Build history of the part. All positions in model axes, mm. A direction names the side the tool comes from. Give positions to 0.01 mm unless a question says otherwise; leave off trailing zeros. Write each loop counter-clockwise with the first axis right and the second up, starting at its lowest first coordinate (ties: lowest second). Pieces come first, ordered by that corner, then holes. Notation, with made-up numbers: M -29,0.5 L -16,0.5 A19 ccw -16,4.5 Z; hole C 84.5,-34 d11. An arc over 180 degrees is marked long. Return JSON: item names as keys, results as strings. Group by question number.
Q1. Band-saw the part on C-C, the plane y = 290. Give the cut face in (x, z) (3 decimals).
Q2. Band-saw the part on A-A, the plane x = -56.5. Give the cut face in (y, z) (3 decimals).
Q3. Pull direction Z, two halves, no side cores. Call faces 1 (the flat face through (-184.15, 279, 100)), 2 (the flat face through (-3, 279, -22.225)), 3 (the flat face through (-190.5, 280, 100)), 4 (the flat face through (-3, 280, 228.6)): +Z half, -Z half, draft (parallel to the pull), parting line (faces both ways), or undercut.
Q4. Tool access for faces 5 (the flat face through (-184.3, 254, 102.2)), 6 (the flat face through (-3, 279, 225.425)): list every direction of +Z, -Z, +X, -X, +Y, -Y with a clear straight run to the whole face (end or side of a thin tool).
Q5. Wall check: probe 1 along Z at (x, y) = (-156, 275) (3 decimals); probe 2 along X at (y, z) = (294, 73.5). Give the ranges that are in metal, low to high.
Q6. Band-saw the part on B-B, the plane z = 58.5. Give the cut face in (x, y).
from build123d import *

# Parameters (mm, degrees)
F0_W     = 381
F0_H     = 254
F1_DEPTH = 50.8
F2_R     = 6.35
F3_R     = 6.35
F5_W     = 368.3
F5_H     = 247.65
F6_DEPTH = 50.8
F7_R     = 3.175


with BuildPart() as f1:
    # F0 (on Front) → F1 (new body)
    with BuildSketch(Plane.XZ):
        Rectangle(F0_W, F0_H)
    extrude(amount=F1_DEPTH)

    # F2
    f2_edges = [f1.edges().sort_by_distance(p)[0] for p in [
        (190.5, -25.4, 127),
    ]]
    fillet(f2_edges, radius=F2_R)

    # F3
    f3_edges = [f1.edges().sort_by_distance(p)[0] for p in [
        (190.5, -25.4, -127),
        (-190.5, -25.4, 127),
        (-190.5, -25.4, -127),
    ]]
    fillet(f3_edges, radius=F3_R)


with BuildPart() as f1_1:
    # F4: moved
    add(f1.part.moved(Location((0, 50.8, 0))))

    # F5 (on Front) → F6 (cut)
    with BuildSketch(Plane.XZ):
        Rectangle(F5_W, F5_H)
    extrude(amount=-F6_DEPTH, mode=Mode.SUBTRACT)

    # F7
    f7_edges = [f1_1.edges().sort_by_distance(p)[0] for p in [
        (184.15, 25.4, -123.825),
        (184.15, 25.4, 123.825),
        (-184.15, 25.4, 123.825),
        (-184.15, 25.4, -123.825),
    ]]
    fillet(f7_edges, radius=F7_R)


with BuildPart() as f1_2:
    # F8: moved
    add(f1_1.part.moved(Location((0, 50.8, 0))))


with BuildPart() as f1_3:
    # F9: moved
    add(f1_2.part.moved(Location((0, 0, -101.6))))


with BuildPart() as f1_4:
    # F10: moved
    add(f1_3.part.moved(Location((0, 203.2, 0))))


with BuildPart() as f1_5:
    # F11: moved
    add(f1_4.part.moved(Location((0, 0, 203.2))))


solid = f1_5.part
From the geometry:
{
 "1": {"outline": "M -190.5,-19.05 A6.35 ccw -184.15,-25.4 L 184.15,-25.4 A6.35 ccw 190.5,-19.05 L 190.5,222.25 A6.35 ccw 184.15,228.6 L -184.15,228.6 A6.35 ccw -190.5,222.25 Z; hole M -184.15,-19.05 A3.175 ccw -180.975,-22.225 L 180.975,-22.225 A3.175 ccw 184.15,-19.05 L 184.15,222.25 A3.175 ccw 180.975,225.425 L -180.975,225.425 A3.175 ccw -184.15,222.25 Z"},
 "2": {"outline": "M 254,-25.4 L 304.8,-25.4 L 304.8,-22.225 L 254,-22.225 Z; M 254,225.425 L 304.8,225.425 L 304.8,228.6 L 254,228.6 Z"},
 "3": {"face 1": "undercut", "face 2": "undercut", "face 3": "draft", "face 4": "+Z half"},
 "4": {"face 5": "+Z, -Z, +X, -X, -Y", "face 6": "+Y, -Y"},
 "5": {"probe 1": "z = -25.4 to -22.225, 225.425 to 228.6", "probe 2": "x = -190.5 to -184.15, 184.15 to 190.5"},
 "6": {"outline": "M -190.5,254 L -184.15,254 L -184.15,304.8 L -190.5,304.8 Z; M 184.15,254 L 190.5,254 L 190.5,304.8 L 184.15,304.8 Z"}
}
